Geometry check sheet. Reference: the model listing, model coordinates, mm. Face numbers are marked on the shaded views. Coordinates: 2 decimals unless noted, no trailing zeros. Write each loop counter-clockwise with the first axis right and the second up, starting at its lowest first coordinate (ties: lowest second). Pieces come first, ordered by that corner, then holes. Notation, with made-up numbers: (27.25, 15.25) -> (31.25, 15.25) arc R13 ccw to (31.25, 26.25) -> close; hole circle Ø11 at (-8, 21). An arc over 180 degrees is marked (long way). One line per question, with ' | ' between items.
```python
from build123d import *

# Parameters (mm, degrees)
SKETCH1_W               = 40.2
SKETCH1_H               = 61.1
BOSS_EXTRUDE1_DEPTH     = 21
CUT_EXTRUDE_THIN1_DEPTH = 42


with BuildPart() as part:
    # Sketch1 → Boss-Extrude1 (new, symmetric)
    with BuildSketch(Plane.XY):
        Rectangle(SKETCH1_W, SKETCH1_H)
    extrude(amount=BOSS_EXTRUDE1_DEPTH, both=True)

    # Sketch2 → Cut-Extrude-Thin1 (cut)
    with BuildSketch(Plane.XY.offset(21)):
        with BuildLine():
            Line((12.43954262, -40.55), (-12.417377754, -40.55))
            ThreePointArc((-12.417377754, -40.55), (-18.882723085, -38.967701468), (-23.886624641, -34.578472821))
            Line((-23.886624641, -34.578472821), (-27.569246887, -29.317583898))
            ThreePointArc((-27.569246887, -29.317583898), (-29.452330441, -25.498062465), (-30.1, -21.289111077))
            Line((-30.1, -21.289111077), (-30.1, 0))
            Line((-30.1, 0), (-30.1, 21.289111077))
            ThreePointArc((-30.1, 21.289111077), (-29.452330441, 25.498062465), (-27.569246887, 29.317583898))
            Line((-27.569246887, 29.317583898), (-23.886624641, 34.578472821))
            ThreePointArc((-23.886624641, 34.578472821), (-18.882723085, 38.967701468), (-12.417377754, 40.55))
            Line((-12.417377754, 40.55), (12.417377754, 40.55))
            ThreePointArc((12.417377754, 40.55), (18.882723085, 38.967701468), (23.886624641, 34.578472821))
            Line((23.886624641, 34.578472821), (27.569246887, 29.317583898))
            ThreePointArc((27.569246887, 29.317583898), (29.452330441, 25.498062465), (30.1, 21.289111077))
            Line((30.1, 21.289111077), (30.1, 0))
            Line((30.1, 0), (30.1, -21.273665037))
            ThreePointArc((30.1, -21.273665037), (29.461154338, -25.454520783), (27.602920748, -29.253816306))
            Line((27.602920748, -29.253816306), (23.942463367, -34.530151269))
            ThreePointArc((23.942463367, -34.530151269), (18.930994007, -38.954074286), (12.43954262, -40.55))
        make_face()
        with BuildLine():
            Line((12.43954262, -30.55), (-12.417377754, -30.55))
            ThreePointArc((-12.417377754, -30.55), (-14.264619277, -30.097914705), (-15.694305436, -28.843849377))
            Line((-15.694305436, -28.843849377), (-19.376927682, -23.582960454))
            ThreePointArc((-19.376927682, -23.582960454), (-19.914951555, -22.491668616), (-20.1, -21.289111077))
            Line((-20.1, -21.289111077), (-20.1, 0))
            Line((-20.1, 0), (-20.1, 21.289111077))
            ThreePointArc((-20.1, 21.289111077), (-19.914951555, 22.491668616), (-19.376927682, 23.582960454))
            Line((-19.376927682, 23.582960454), (-15.694305436, 28.843849377))
            ThreePointArc((-15.694305436, 28.843849377), (-14.264619277, 30.097914705), (-12.417377754, 30.55))
            Line((-12.417377754, 30.55), (12.417377754, 30.55))
            ThreePointArc((12.417377754, 30.55), (14.264619277, 30.097914705), (15.694305436, 28.843849377))
            Line((15.694305436, 28.843849377), (19.376927682, 23.582960454))
            ThreePointArc((19.376927682, 23.582960454), (19.914951555, 22.491668616), (20.1, 21.289111077))
            Line((20.1, 21.289111077), (20.1, 0))
            Line((20.1, 0), (20.1, -21.273665037))
            ThreePointArc((20.1, -21.273665037), (19.917472668, -22.46819525), (19.386548785, -23.553708257))
            Line((19.386548785, -23.553708257), (15.726091405, -28.83004322))
            ThreePointArc((15.726091405, -28.83004322), (14.294243016, -30.094021224), (12.43954262, -30.55))
        make_face(mode=Mode.SUBTRACT)
    extrude(amount=-CUT_EXTRUDE_THIN1_DEPTH, mode=Mode.SUBTRACT)


solid = part.part
```
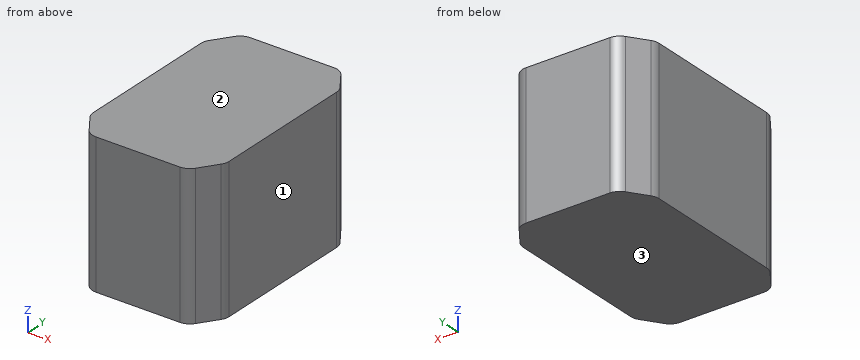
(1) Cross-section at B-B (x = -16.5). Record the cut outline in (y, z), plus the area to 3 significant figures.
Answers below:
outline: (-27.69, -21) -> (27.69, -21) -> (27.69, 21) -> (-27.69, 21) -> close | area: 2,330 mm²
(2) Draft check along Z on the marked faces 1, 2 and 3. Enter one of: pulls with the +Z half, pulls with the -Z half, needs draft (parallel to the pull), parting line crosses it, or undercut.
Answers below:
face 1: needs draft | face 2: pulls with the +Z half | face 3: pulls with the -Z half
(3) Cross-section at A-A (z = -1.5). Record the cut outline in (x, y), plus the area to 3 significant figures.
Answers below:
outline: (-20.1, -21.29) arc R4 ccw to (-19.38, -23.58) -> (-15.69, -28.84) arc R4 ccw to (-12.42, -30.55) -> (12.44, -30.55) arc R4 ccw to (15.73, -28.83) -> (19.39, -23.55) arc R4 ccw to (20.1, -21.27) -> (20.1, 21.29) arc R4 ccw to (19.38, 23.58) -> (15.69, 28.84) arc R4 ccw to (12.42, 30.55) -> (-12.42, 30.55) arc R4 ccw to (-15.69, 28.84) -> (-19.38, 23.58) arc R4 ccw to (-20.1, 21.29) -> close | area: 2,360 mm²
(4) Material ranges on line 1 (Y direction, x = 18.5, z = 0.5); line 2 (Y direction, x = 15, z = 11); line 3 (X direction, y = 25, z = 4) (3 decimals), recorded low to high.
Answers below:
line 1: y = -24.83 to 24.84 | line 2: y = -29.62 to 29.6 | line 3: x = -18.385 to 18.385
